from build123d import *

# Parameters (mm, degrees)
BOSS_EXTRU_1_DEPTH = 3
CONG_1_R           = 100


with BuildPart() as part:
    # Esquisse1 → Boss.-Extru.1 (new body)
    with BuildSketch(Plane.XY):
        Polygon((-103.923413348, 35.431604979), (176.076586652, 35.431604979), (166.152848879, -10.376473534), (68.721994761, -26.257415358), (40.576586652, -27.568395021), (40.576586652, -17.368395021), (31.576586652, -17.368395021), (31.576586652, -27.568395021), (3.431178543, -26.257415358), (-93.999675575, -10.376473534), align=None)
    extrude(amount=BOSS_EXTRU_1_DEPTH)

    # Congé1
    # the kernel refuses this fillet: 100 mm, written as the material it takes off along each edge
    with BuildSketch(Plane(origin=(166.152848879, -10.376473534, -163.559702543), x_dir=(0.21172591921769693, 0.9773290823112863, 0), z_dir=(0, 0, 1))) as cong_1_piece_1:
        with BuildLine():
            CenterArc((69.095913034, 97.498917991), CONG_1_R, 201.481144987, 55.677497197)
            Line((-23.957899624, 60.879415675), (-25.818975877, 60.147025629))
            Line((-25.818975877, 60.147025629), (-1.861076253, -0.732390046))
            Line((-1.861076253, -0.732390046), (0, -2))
            ThreePointArc((0, -2), (23.435339919, -2), (46.426175173, -1.94997836))
            Line((46.426175173, -1.94997836), (46.870679837, 0))
        make_face()
    extrude(amount=330.119405086, mode=Mode.SUBTRACT)
    with BuildSketch(Plane(origin=(68.721994761, -26.257415358, -14.394746153), x_dir=(0.9869749511957248, 0.16087400570694135, 0), z_dir=(0, 0, 1)), Plane(origin=(3.431178543, -26.257415358, -14.394746153), x_dir=(0.9989169691295284, -0.04652836538152723, 0), z_dir=(0, 0, 1))) as cong_1_piece_2:
        with BuildLine():
            CenterArc((CONG_1_R * 0.057578984614, CONG_1_R), CONG_1_R, 263.409211525, 6.590788475)
            Line((-CONG_1_R * 0.0571984584269, CONG_1_R * 0.00660876862688), (-CONG_1_R * 0.0594940072877, -CONG_1_R * 0.0132590560006))
            Line((-CONG_1_R * 0.0594940072877, -CONG_1_R * 0.0132590560006), (-CONG_1_R * 0.00115157969228, -CONG_1_R * 0.02))
            Line((-CONG_1_R * 0.00115157969228, -CONG_1_R * 0.02), (CONG_1_R * 0.057578984614, -CONG_1_R * 0.02))
            Line((CONG_1_R * 0.057578984614, -CONG_1_R * 0.02), (CONG_1_R * 0.057578984614, 0))
        make_face()
    extrude(amount=31.789492307, mode=Mode.SUBTRACT)
    with BuildSketch(Plane(origin=(-93.999675575, -10.376473534, -163.559702543), x_dir=(0.9869749511957245, -0.1608740057069428, 0), z_dir=(0, 0, 1))) as cong_1_piece_3:
        with BuildLine():
            CenterArc((65.423881017, 100), CONG_1_R, 214.322502803, 55.677497197)
            Line((-17.163809688, 43.614954607), (-18.815563502, 42.487253699))
            ThreePointArc((-18.815563502, 42.487253699), (-10.442981097, 21.075087257), (-1.861076253, -0.732390046))
            Line((-1.861076253, -0.732390046), (0, -2))
            Line((0, -2), (65.423881017, -2))
            Line((65.423881017, -2), (65.423881017, 0))
        make_face()
    extrude(amount=330.119405086, mode=Mode.SUBTRACT)


solid = part.part
CAD build for the part. Positions are in the model's coordinates, mm. Round coordinates to 2 decimals unless told otherwise and drop trailing zeros. Order: outer loops, then holes, each group sorted by start corner. A loop starts at its lowest first (then second) coordinate and runs counter-clockwise, first axis right, second up. Notation, with made-up numbers: (63, 51) -> (71, 51) arc R27 ccw to (71, 71) -> close; hole circle Ø8 at (-28, -34.75). An arc over 180 degrees is marked (long way). Write each question's results on one line, items separated by ' | '.
1. Cut at A-A (z = 0.75). Give the cut face in (x, y).
Findings below:
outline: (-103.92, 35.43) arc R100 ccw to (-29.43, -20.9) -> (-2.25, -25.33) arc R100 ccw to (9.18, -26.53) -> (31.58, -27.57) -> (31.58, -17.37) -> (40.58, -17.37) -> (40.58, -27.57) -> (62.97, -26.53) arc R100 ccw to (74.4, -25.33) -> (101.58, -20.9) arc R100 ccw to (176.08, 35.43) -> close
2. Wall check: line 1 along X through (y, z) = (25.5, 1.5); line 2 along X through (y, z) = (24, 2.65); line 3 along Y through (x, z) = (-69.5, 1). Give the ranges that are in metal, low to high. Write a range as [from, to].
Findings below:
line 1: x = [-98.58, 170.73] | line 2: x = [-97.64, 169.79] | line 3: y = [-4.95, 35.43]
3. Cut at B-B (x = 157). Give the cut face in (y, z).
Findings below:
outline: (7.89, 0) -> (35.43, 0) -> (35.43, 3) -> (7.89, 3) -> close
4. Flat gauge pins, fed straight in: P1, Ø5, axis at x = 78.5, y = -1.5, coming from the -Z side; P2, Ø1.5, axis at x = -52.5, z = 1.5, coming from the -Y side; P3, Ø1.5, axis at x = 37, z = 2, coming from the -Y side. Where does each tip first touch, or does it go through?
Findings below:
P1: stops at z = 0 | P2: stops at y = -14.53 | P3: stops at y = -17.37
5. Cut at C-C (y = -4). Give the cut face in (x, z), plus the area to 3 significant figures.
Findings below:
outline: (-70.87, 0) -> (143.02, 0) -> (143.02, 3) -> (-70.87, 3) -> close | area: 642 mm²
